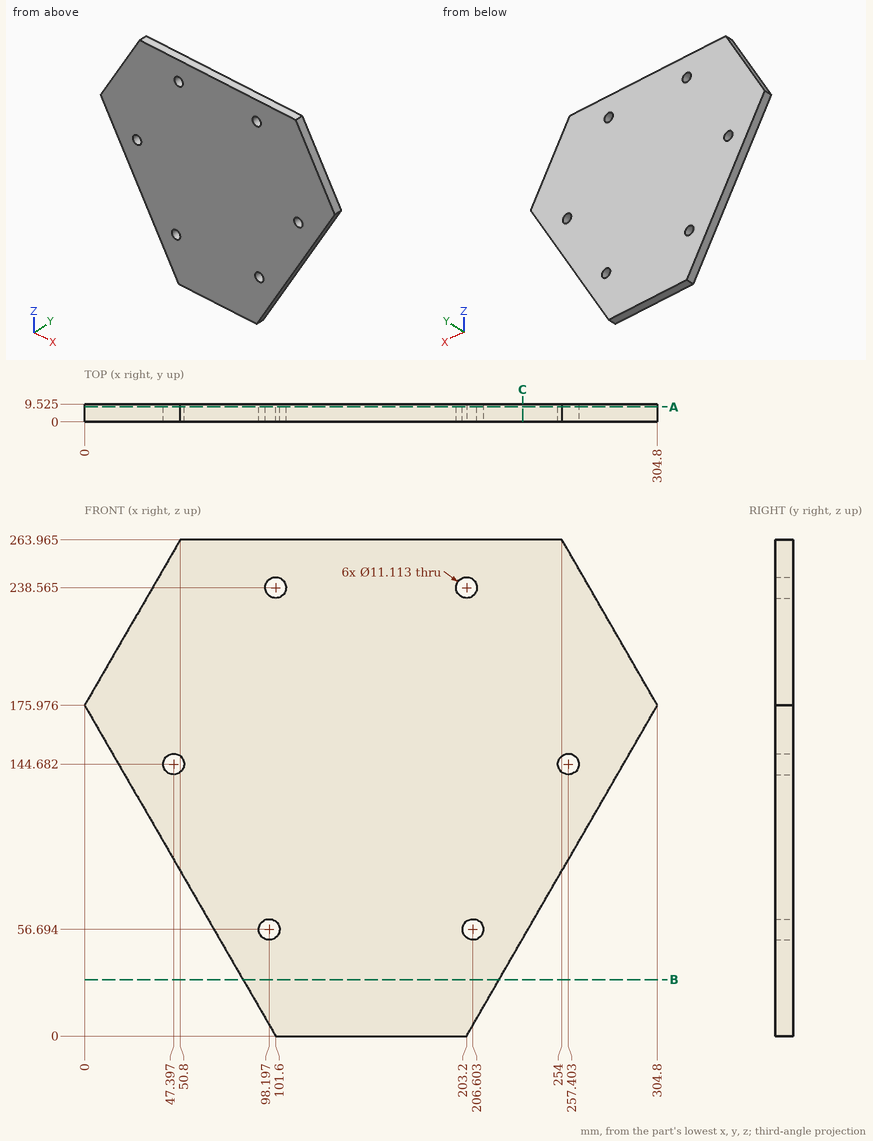
Source: three-view drawing plus pictorial views. Frame: mm from the lowest corner of the part. Coordinates: 2 decimals unless noted, no trailing zeros. Order: outer loops, then holes, each group sorted by start corner. A loop starts at its lowest first (then second) coordinate and runs counter-clockwise, first axis right, second up. Notation, with made-up numbers: M 48,80.5 L 97,80.5 A19 ccw 97,86.5 Z; hole C -23,0.5 d11. An arc over 180 degrees is marked long. Write each question's results on one line, items separated by ' | '. Start each with the question number.
1. Pin query (flat end, axial travel): pin 1 (2 mm diameter, centred on y = 6.5, z = 39.5, fed in from +X); pin 2 (1 mm diameter, centred on x = 264.5, y = 6, fed in from +Z) (1 decimal); pin 3 (1.5 mm diameter, centred on y = 1, z = 219.5, fed in from -X) (1 decimal). Return the tip coordinate at first contact, or that it passes through.
2. Section A-A, the plane y = 8. Return the cut outline in (x, z) (1 decimal), then the cut area to 3 significant figures.
3. Section B-B, the plane z = 30. Return the cut outline in (x, y) (1 decimal).
4. Section C-C, the plane x = 233. Return the cut outline in (y, z) (1 decimal), then the cut area to 3 significant figures.
5. Material intervals for L1, parallel to Z at x = 203.2, y = 2 (1 decimal); L2, parallel to X at y = 3.5, z = 160 (1 decimal); L3, parallel to X at y = 8.25, z = 50, sorted ascending.
Solution:
1) pin 1: x = 226.58 | pin 2: z = 246.6 | pin 3: x = 24.7
2) outline: M 0,176 L 101.6,0 L 203.2,0 L 304.8,176 L 254,264 L 50.8,264 Z; hole C 47.4,144.7 d11.1; hole C 98.2,56.7 d11.1; hole C 101.6,238.6 d11.1; hole C 203.2,238.6 d11.1; hole C 206.6,56.7 d11.1; hole C 257.4,144.7 d11.1 | area: 57,500 mm²
3) outline: M 84.3,0 L 220.5,0 L 220.5,9.5 L 84.3,9.5 Z
4) outline: M 0,51.6 L 9.5,51.6 L 9.5,264 L 0,264 Z | area: 2,020 mm²
5) L1: 0 to 52.3, 61.1 to 233, 244.1 to 264 | L2: 9.2 to 295.6 | L3: 72.73 to 232.07
